Autodesk Inventor part; units mm, degrees
ref_plane "YZ Plane" through (0, 0, 0) normal (1, 0, 0) x (0, 1, 0)
ref_plane "XZ Plane" through (0, 0, 0) normal (0, 1, 0) x (-1, 0, 0)
ref_plane "XY Plane" through (0, 0, 0) normal (0, 0, 1) x (1, 0, 0)
sketch "Sketch1" plane through (0, 0, 0) normal (0, 1, 0) x (-1, 0, 0)
  line L0 (0, 0) -> (-20, 0)
  line L1 (-20, 0) -> (-20, -40.3)
  line L2 (-20, -40.3) -> (0, -40.3)
  line L3 (0, -40.3) -> (0, 0)
  dimension "d0" = 20
  dimension "d1" = 40.3
extrude "Extrusion1" add sketch "Sketch1" along normal blind 36.6
fillet "Fillet1" radius 2 4 edges at (20, 18.3, 0) (0, 18.3, 0) (20, 18.3, -40.3) (0, 18.3, -40.3)
chamfer "Chamfer1" distance 2 angle 45 8 edges at (20, 0, -20.15) (19.4142, 0, -39.7142) (10, 0, -40.3) (0.5858, 0, -39.7142) (0, 0, -20.15) (0.5858, 0, -0.5858) (10, 0, 0) (19.4142, 0, -0.5858)
fillet "Fillet2" radius 1 8 edges at (19.4142, 36.6, -39.7142) (10, 36.6, -40.3) (0.5858, 36.6, -39.7142) (0, 36.6, -20.15) (0.5858, 36.6, -0.5858) (10, 36.6, 0) (19.4142, 36.6, -0.5858) (20, 36.6, -20.15)
sketch "Sketch2" plane through (0, 36.6, 0) normal (0, 1, 0) x (1, 0, 0)
  line L0 (2, 0) -> (18, 0)
  line L1 (18, 0) -> (2, 0)
  line L2 (10, 0) -> (10, 33.5)
  line L3 (10, 0) -> (43.5, 0) construction
  circle A0 centre (10, 33.5) radius 3
  point P0 (0, 0)
  dimension "d9" = 33.5
  dimension "d10" = 90
  dimension "d11" = 6
extrude "Extrusion2" add sketch "Sketch2" along normal blind 5
sketch "Sketch3" plane through (2, 2, 0) normal (0, 0, 1) x (1, 0, 0)
  line L0 (0, -2) -> (16, -2)
  line L1 (18, 33.6) -> (18, 0)
  line L2 (-2, 27.6) -> (18, 27.6)
  line L3 (18, 27.6) -> (18, 24.6)
  line L4 (18, 24.6) -> (-2, 24.6)
  line L5 (-2, 24.6) -> (-2, 27.6)
  point P0 (-2, -2)
  dimension "d14" = 3
  dimension "d15" = 26.6
extrude "Extrusion3" add sketch "Sketch3" along normal blind 6.65 and the other way blind 46.95
fillet "Fillet3" radius 1 4 edges at (20, 28.1, 6.65) (0, 28.1, 6.65) (20, 28.1, -46.95) (0, 28.1, -46.95)
properties part number "Servo"
Read the model definition and answer for the solid it produces. Units are mm, in the model's axes. A direction names the side the tool comes from. Give positions to 0.01 mm unless a question says otherwise; leave off trailing zeros. Loops run counter-clockwise (first coordinate to the right, second up) from the corner with the lowest first, then second, coordinate; pieces in that order, holes last. Notation, with made-up numbers: (-1.75, 86) -> (22.25, 86) arc R8 ccw to (22.25, 93) -> close; hole circle Ø9 at (-18, -5). An arc over 180 degrees is marked (long way). Answer as CSV lines item,"result".
Item 1: Find section D-D on x = 10. Give the vertices of the cut face in (y, z).
Returned:
outline,"(0, -38.3) -> (2, -40.3) -> (26.6, -40.3) -> (26.6, -46.95) -> (29.6, -46.95) -> (29.6, -40.3) -> (35.6, -40.3) arc R1 ccw to (36.6, -39.3) -> (36.6, -36.5) -> (41.6, -36.5) -> (41.6, -30.5) -> (36.6, -30.5) -> (36.6, -1) arc R1 ccw to (35.6, 0) -> (29.6, 0) -> (29.6, 6.65) -> (26.6, 6.65) -> (26.6, 0) -> (2, 0) -> (0, -2) -> close"
Item 2: Find section C-C on z = -33.5. Give the vertices of the cut face in (x, y), plus the area to 3 significant figures.
Returned:
outline,"(0, 2) -> (2, 0) -> (18, 0) -> (20, 2) -> (20, 35.6) arc R1 ccw to (19, 36.6) -> (13, 36.6) -> (13, 41.6) -> (7, 41.6) -> (7, 36.6) -> (1, 36.6) arc R1 ccw to (0, 35.6) -> close"
area,"758 mm²"
Item 3: Consider line 1 (Y direction, x = 2, z = -36.5); line 2 (Z direction, x = 14, y = 14); line 3 (Y direction, x = 5.5, z = -42.5). Determine where each line is inside the solid, lowest interval first. Write a range as [from, to].
Returned:
line 1,"y = [0, 36.6]"
line 2,"z = [-40.3, 0]"
line 3,"y = [26.6, 29.6]"
Item 4: Each of these flat-tipped pins is pushed along its axis until it touches: pin 1 (5 mm diameter, centred on x = 12.5, y = 32.5, fed in from +Z); pin 2 (1 mm diameter, centred on x = 16, y = 13, fed in from -Z); pin 3 (5 mm diameter, centred on x = 15, z = -41, fed in from -Y). Where does it stop, or does it pass through?
Returned:
pin 1,"stops at z = 0"
pin 2,"stops at z = -40.3"
pin 3,"stops at y = 0.2"
Item 5: For faces 1 (the face through (10, 14, 0)), 2 (the face through (10, 33, -40.3)), 3 (the face through (19.43, 14.47, -39.7)), 4 (the face through (0.6, 14.47, -39.73)), determine the directions among +Z, -Z, +X, -X, +Y, -Y from which every point of the face is accessible in a straight line to the end or side of a thin tool.
Returned:
face 1,"+Z, +X, -X, -Y"
face 2,"-Z, +X, -X, +Y"
face 3,"-Z, +X, -Y"
face 4,"-Z, -X, -Y"
Item 6: Determine the mould class of faces 5 (the face through (10, 0, -20)), 6 (the face through (10, 1, -1)), 7 (the face through (10.1, 1, -39.3)) for opening direction Z: +Z half, -Z half, draft (parallel to the pull), parting line (faces both ways), or undercut.
Returned:
face 5,"draft"
face 6,"+Z half"
face 7,"-Z half"
Item 7: Find section A-A on x = 16. Give the vertices of the cut face in (y, z), plus the area to 3 significant figures.
Returned:
outline,"(0, -38.3) -> (2, -40.3) -> (26.6, -40.3) -> (26.6, -46.95) -> (29.6, -46.95) -> (29.6, -40.3) -> (35.6, -40.3) arc R1 ccw to (36.6, -39.3) -> (36.6, -1) arc R1 ccw to (35.6, 0) -> (29.6, 0) -> (29.6, 6.65) -> (26.6, 6.65) -> (26.6, 0) -> (2, 0) -> (0, -2) -> close"
area,"1,510 mm²"
Item 8: Find section B-B on y = 9. Give the vertices of the cut face in (x, z).
Returned:
outline,"(0, -38.3) arc R2 ccw to (2, -40.3) -> (18, -40.3) arc R2 ccw to (20, -38.3) -> (20, -2) arc R2 ccw to (18, 0) -> (2, 0) arc R2 ccw to (0, -2) -> close"
